Read the model definition and answer for the solid it produces. Units are mm, in the model's axes. Face numbers are marked on the shaded views. A direction names the side the tool comes from. Round coordinates to 2 decimals unless told otherwise and drop trailing zeros. Loops run counter-clockwise (first coordinate to the right, second up) from the corner with the lowest first, then second, coordinate; pieces in that order, holes last. Notation, with made-up numbers: M -32.75,0.5 L -18.75,0.5 A27 ccw -18.75,20.5 Z; hole C -17.5,-34.75 d5. An arc over 180 degrees is marked long. Answer as CSV lines item,"result".
```python
from build123d import *

# Parameters (mm, degrees)
SKETCH1_W           = 25.4
SKETCH1_H           = 38.1
BOSS_EXTRUDE1_DEPTH = 4.75
SKETCH2_W           = 3.4
SKETCH2_H           = 30.1
CUT_EXTRUDE1_DEPTH  = 24.382792819
FILLET1_R           = 1.7
FILLET2_R           = 1.7
FILLET3_R           = 1.7
FILLET4_R           = 1.7
FILLET5_R           = 2
FILLET6_R           = 1.7
FILLET7_R           = 1.7


with BuildPart() as part:
    # Sketch1 → Boss-Extrude1 (new body)
    with BuildSketch(Plane.XY):
        Rectangle(SKETCH1_W, SKETCH1_H)
    extrude(amount=BOSS_EXTRUDE1_DEPTH)

    # Sketch2 → Cut-Extrude1 (cut, through all)
    with BuildSketch(Plane.XY.offset(4.75)):
        with Locations((7.5, 0)):
            Rectangle(SKETCH2_W, SKETCH2_H)
        with Locations((-7.5, 0)):
            Rectangle(SKETCH2_W, SKETCH2_H)
        Rectangle(SKETCH2_W, SKETCH2_H)
    extrude(amount=-CUT_EXTRUDE1_DEPTH, mode=Mode.SUBTRACT)

    # Fillet1
    fillet1_edges = [part.edges().sort_by_distance(p)[0] for p in [
        (-5.8, 15.05, 2.375),
        (-9.2, 15.05, 2.375),
    ]]
    fillet(fillet1_edges, radius=FILLET1_R - 0.0001)  # a hair under: the kernel refuses the full size

    # Fillet2
    fillet2_edges = [part.edges().sort_by_distance(p)[0] for p in [
        (-5.8, -15.05, 2.375),
        (-9.2, -15.05, 2.375),
    ]]
    fillet(fillet2_edges, radius=FILLET2_R - 0.0001)  # a hair under: the kernel refuses the full size

    # Fillet3
    fillet3_edges = [part.edges().sort_by_distance(p)[0] for p in [
        (9.2, 15.05, 2.375),
        (5.8, 15.05, 2.375),
    ]]
    fillet(fillet3_edges, radius=FILLET3_R - 0.0001)  # a hair under: the kernel refuses the full size

    # Fillet4
    fillet4_edges = [part.edges().sort_by_distance(p)[0] for p in [
        (9.2, -15.05, 2.375),
        (5.8, -15.05, 2.375),
    ]]
    fillet(fillet4_edges, radius=FILLET4_R - 0.0001)  # a hair under: the kernel refuses the full size

    # Fillet5
    fillet5_edges = [part.edges().sort_by_distance(p)[0] for p in [
        (-12.7, 0, 4.75),
        (0, -19.05, 4.75),
        (12.7, 0, 4.75),
        (0, -19.05, 0),
        (-12.7, 0, 0),
        (12.7, 0, 0),
        (12.7, -19.05, 2.375),
        (-12.7, -19.05, 2.375),
    ]]
    fillet(fillet5_edges, radius=FILLET5_R)

    # Fillet6
    fillet6_edges = [part.edges().sort_by_distance(p)[0] for p in [
        (1.7, 15.05, 2.375),
        (-1.7, 15.05, 2.375),
    ]]
    fillet(fillet6_edges, radius=FILLET6_R - 0.0001)  # a hair under: the kernel refuses the full size

    # Fillet7
    fillet7_edges = [part.edges().sort_by_distance(p)[0] for p in [
        (1.7, -15.05, 2.375),
        (-1.7, -15.05, 2.375),
    ]]
    fillet(fillet7_edges, radius=FILLET7_R - 0.0001)  # a hair under: the kernel refuses the full size


solid = part.part
```
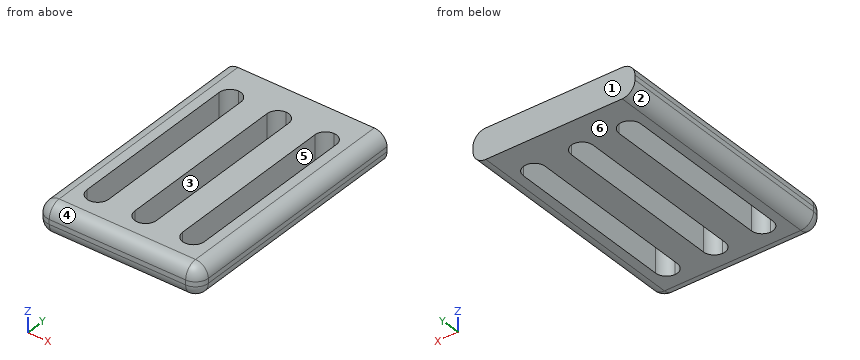
1) Find section A-A, the plane y = 12. Give the vertices of the cut face in (x, z).
Evaluation:
outline,"M -12.7,2 A2 ccw -10.7,0 L -9.2,0 L -9.2,4.75 L -10.7,4.75 A2 ccw -12.7,2.75 Z; M -5.8,0 L -1.7,0 L -1.7,4.75 L -5.8,4.75 Z; M 1.7,0 L 5.8,0 L 5.8,4.75 L 1.7,4.75 Z; M 9.2,0 L 10.7,0 A2 ccw 12.7,2 L 12.7,2.75 A2 ccw 10.7,4.75 L 9.2,4.75 Z"
2) Straight lines are drawn through the part: line 1 (X direction, y = -6, z = 2.85); line 2 (X direction, y = 7, z = 3.2); line 3 (Y direction, x = -6.5, z = 3.95). For each, find the intervals that lie inside material, in ascending order.
Evaluation:
line 1,"x = -12.7 to -9.2, -5.8 to -1.7, 1.7 to 5.8, 9.2 to 12.7"
line 2,"x = -12.65 to -9.2, -5.8 to -1.7, 1.7 to 5.8, 9.2 to 12.65"
line 3,"y = -18.65 to -14.72, 14.72 to 19.05"
3) Determine the mould class of the marked faces 1, 2, 3 and 4 for opening direction Y: released by +Y, released by -Y, zero draft, split by the parting line, or undercut.
Evaluation:
face 1,"released by +Y"
face 2,"zero draft"
face 3,"undercut"
face 4,"released by -Y"
4) Find section B-B, the plane x = 8.25. Give the vertices of the cut face in (y, z).
Evaluation:
outline,"M -19.05,2 A2 ccw -17.05,0 L -14.88,0 L -14.88,4.75 L -17.05,4.75 A2 ccw -19.05,2.75 Z; M 14.88,0 L 19.05,0 L 19.05,4.75 L 14.88,4.75 Z"
5) Find section D-D, the plane z = 3.4. Count the separate pieces of the cut face and the enclosed holes in it, then the cut area to 3 significant figures.
Evaluation:
separate pieces,"1"
enclosed holes,"3"
area,"656 mm^2"
6) A tool of negligible diameter and unlimited length cuts with its end or side. For the marked faces 5 and 6, from which of +Z, -Z, +X, -X, +Y, -Y can it reach the whole face along a straight path? Write none if from no direction.
Evaluation:
face 5,"+Z, -Z"
face 6,"-Z, +X, -X, +Y, -Y"
7) Each of these flat-tipped pins is pushed along its axis until it touches: P1, Ø1.4, axis at y = 0, z = 3.5, coming from the -X side; P2, Ø1.5, axis at y = -11.5, z = 4, coming from the +X side; P3, Ø1.5, axis at x = 0.5, y = -4.5, coming from the +Z side; P4, Ø1.5, axis at x = 8.5, z = 4, coming from the -Y side. Where does it stop, or does it pass through?
Evaluation:
P1,"stops at x = -12.7"
P2,"stops at x = 12.64"
P3,"passes through"
P4,"stops at y = -18.99"
8) Find section C-C, the plane y = -16. Give the vertices of the cut face in (x, z), then the cut area to 3 significant figures.
Evaluation:
outline,"M -12.7,2 A2 ccw -10.7,0 L 10.7,0 A2 ccw 12.7,2 L 12.7,2.75 A2 ccw 10.7,4.75 L -10.7,4.75 A2 ccw -12.7,2.75 Z"
area,"117 mm^2"
